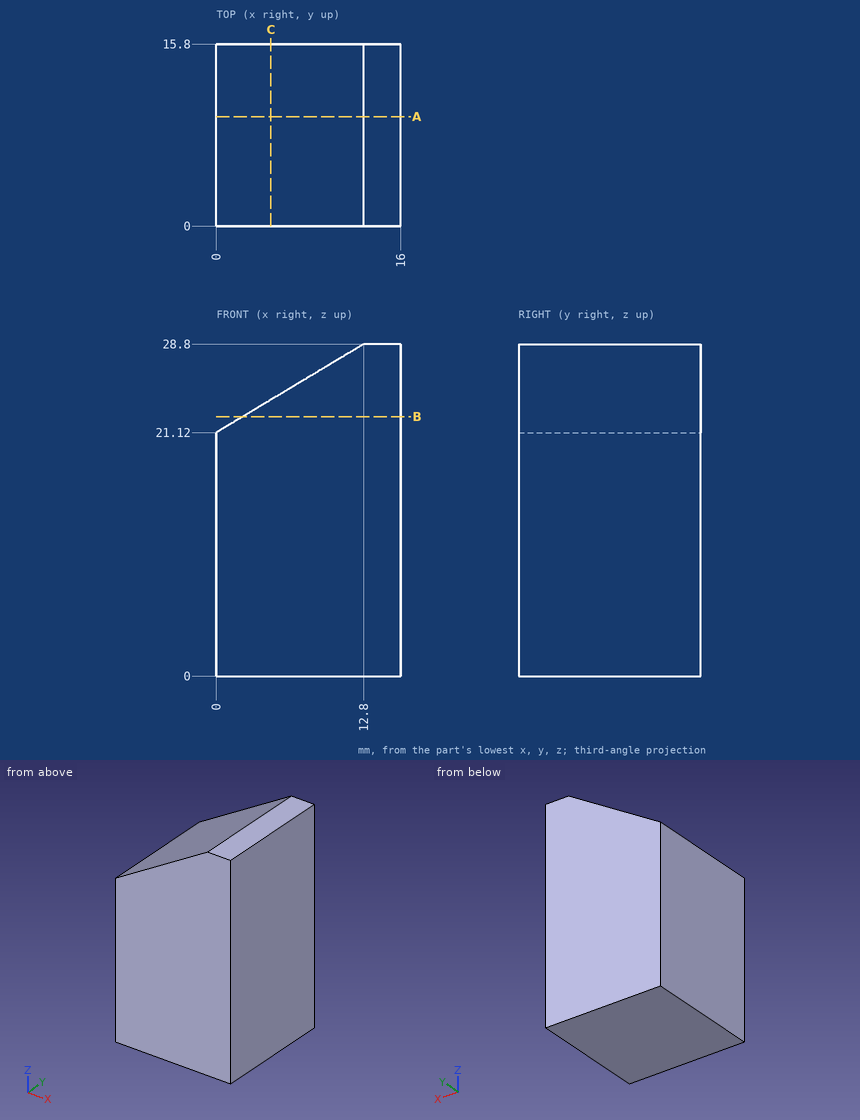
For this review, use the dimensioned drawing (mm, ordinates from the lowest corner) and the shaded views. Give positions to 0.01 mm unless a question says otherwise; leave off trailing zeros. Order: outer loops, then holes, each group sorted by start corner. A loop starts at its lowest first (then second) coordinate and runs counter-clockwise, first axis right, second up.
1) Take a section at A-A (y = 9.5). Give the boundary of the cut face in (x, z), then the cut area to 3 significant figures.
2) Wall thickness on line 1 (X direction, y = 5.25, z = 24.5); line 2 (Z direction, x = 10.5, y = 13.75); line 3 (Z direction, x = 6.5, y = 0.5): over which ranges is each line inside the solid? List them lowest first.
3) Take a section at C-C (x = 4.75). Give the boundary of the cut face in (y, z), then the cut area to 3 significant figures.
4) Take a section at B-B (z = 22.5). Give the boundary of the cut face in (x, y), then the cut area to 3 significant figures.
Derived:
1. outline: (0, 0) - (16, 0) - (16, 28.8) - (12.8, 28.8) - (0, 21.12) - close
1. area: 412 mm2
2. line 1: x = 5.63 to 16
2. line 2: z = 0 to 27.42
2. line 3: z = 0 to 25.02
3. outline: (0, 0) - (15.8, 0) - (15.8, 23.97) - (0, 23.97) - close
3. area: 379 mm2
4. outline: (2.3, 0) - (16, 0) - (16, 15.8) - (2.3, 15.8) - close
4. area: 216 mm2
